For this review, take the finished solid that the model builds, in its own axes (mm). Face numbers are marked on the shaded views. A direction names the side the tool comes from. Coordinates: 2 decimals unless noted, no trailing zeros. Order: outer loops, then holes, each group sorted by start corner. A loop starts at its lowest first (then second) coordinate and runs counter-clockwise, first axis right, second up. Notation, with made-up numbers: (-21, -23.75) -> (5, -23.75) arc R23 ccw to (5, 8.25) -> close; hole circle Ø10 at (-1, -32). An arc over 180 degrees is marked (long way). Answer as a JSON object with one key per item and string values. Group by question number.
1) Add section C-C, the plane y = -7.5. Write out the cut boundary in (x, z).
2) Add section A-A, the plane z = 12. Write out the cut boundary in (x, y).
3) Draft analysis for pull direction Z (two halves, no side actions). For the marked faces 1, 2 and 3, state which applies: +Z half, -Z half, draft (parallel to the pull), parting line (faces both ways), or undercut.
4) Add section B-B, the plane x = 0.5. Write out the cut boundary in (y, z).
5) Wall thickness on L1, parallel to X at y = -7.75, z = -8; L2, parallel to Z at x = -1.5, y = -4.75; L3, parallel to Z at x = 9.25, y = -3.5: over which ranges is each line inside the solid? List them lowest first.
6) For pin 1 (6 mm diameter, centred on x = -7.5, z = -8.5, fed in from +Y); pin 2 (8 mm diameter, centred on x = -3, z = -14, fed in from -Y), all flat-tipped, find the tip position at first contact; note any pin that passes through.
7) Machinability: for the marked faces 4 and 5, which of the approach directions +Z, -Z, +X, -X, +Y, -Y give a long, thin tool a straight path to every point of the face, cutting with its end or side? Answer none if there is none.
from build123d import *

# Parameters (mm, degrees)
BASES_W            = 19.8
BASES_H            = 40.6
BASE_DEPTH         = 10.25
BASE_F_R           = 1
CUT_EXTRUDE3_DEPTH = 21.5


with BuildPart() as part:
    # BaseS → BASE (new body, symmetric)
    with BuildSketch(Plane(origin=(0, 0, 0), x_dir=(1, 0, 0), z_dir=(0, 1, 0))):
        Rectangle(BASES_W, BASES_H)
    extrude(amount=BASE_DEPTH, both=True)

    # BASE F
    base_f_edges = [part.edges().sort_by_distance(p)[0] for p in [
        (9.9, 0, 20.3),
        (-9.9, 0, 20.3),
        (-9.9, 0, -20.3),
        (9.9, 0, -20.3),
    ]]
    fillet(base_f_edges, radius=BASE_F_R)

    # PocketS → Cut-Extrude3 (cut, through all)
    with BuildSketch(Plane(origin=(0, 10.25, 0), x_dir=(1, 0, 0), z_dir=(0, 1, 0))):
        with BuildLine():
            Line((8.9, 19.5), (-8.9, 19.5))
            ThreePointArc((-8.9, 19.5), (-9.041421356, 19.441421356), (-9.1, 19.3))
            Line((-9.1, 19.3), (-9.1, -19.3))
            ThreePointArc((-9.1, -19.3), (-9.041421356, -19.441421356), (-8.9, -19.5))
            Line((-8.9, -19.5), (8.9, -19.5))
            ThreePointArc((8.9, -19.5), (9.041421356, -19.441421356), (9.1, -19.3))
            Line((9.1, -19.3), (9.1, 19.3))
            ThreePointArc((9.1, 19.3), (9.041421356, 19.441421356), (8.9, 19.5))
        make_face()
    extrude(amount=-CUT_EXTRUDE3_DEPTH, mode=Mode.SUBTRACT)


solid = part.part
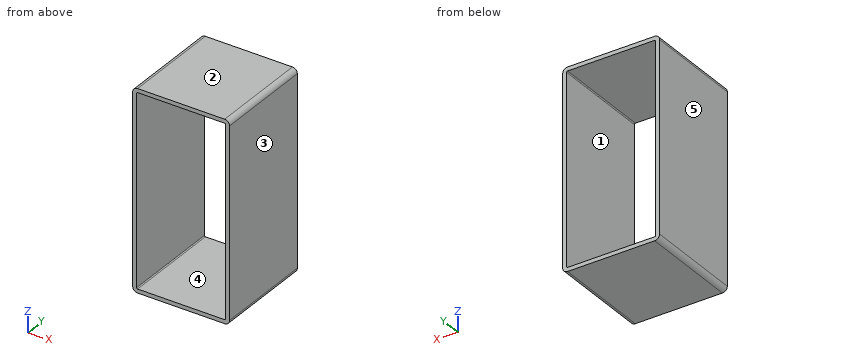
Output values:
{
 "1": {"outline": "(-9.9, -19.3) arc R1 ccw to (-8.9, -20.3) -> (8.9, -20.3) arc R1 ccw to (9.9, -19.3) -> (9.9, 19.3) arc R1 ccw to (8.9, 20.3) -> (-8.9, 20.3) arc R1 ccw to (-9.9, 19.3) -> close; hole (-9.1, -19.3) arc R0.2 ccw to (-8.9, -19.5) -> (8.9, -19.5) arc R0.2 ccw to (9.1, -19.3) -> (9.1, 19.3) arc R0.2 ccw to (8.9, 19.5) -> (-8.9, 19.5) arc R0.2 ccw to (-9.1, 19.3) -> close"},
 "2": {"outline": "(-9.9, -10.25) -> (-9.1, -10.25) -> (-9.1, 10.25) -> (-9.9, 10.25) -> close; (9.1, -10.25) -> (9.9, -10.25) -> (9.9, 10.25) -> (9.1, 10.25) -> close"},
 "3": {"face 1": "undercut", "face 2": "+Z half", "face 3": "draft"},
 "4": {"outline": "(-10.25, -20.3) -> (10.25, -20.3) -> (10.25, -19.5) -> (-10.25, -19.5) -> close; (-10.25, 19.5) -> (10.25, 19.5) -> (10.25, 20.3) -> (-10.25, 20.3) -> close"},
 "5": {"L1": "x = -9.9 to -9.1, 9.1 to 9.9", "L2": "z = -20.3 to -19.5, 19.5 to 20.3", "L3": "z = -20.24 to 20.24"},
 "6": {"pin 1": "stops at y = 10.25", "pin 2": "passes through"},
 "7": {"face 4": "+Y, -Y", "face 5": "+Z, -Z, -X, +Y, -Y"}
}
